Could you check a few things on this model? Use its own coordinates, in mm. Give positions to 0.01 mm unless a question says otherwise; leave off trailing zeros. Loops run counter-clockwise (first coordinate to the right, second up) from the corner with the lowest first, then second, coordinate; pieces in that order, holes last.
1. Imagine slicing it at A-A (y = -4.5). Count the separate pieces of the cut face and the enclosed holes in it, plus the area to 3 significant figures.
2. For P1, Ø18, axis at x = 0, z = 185, coming from the +Y side, with a flat end and sliding along its axis, tell me the tip position at first contact or that it passes through.
3. Thinking about a two-plate mould opening in Z: for faces 1 (the cylindrical face through (-1.302, 0.858, 94.915)), 2 (the cylindrical face through (-2.17, 0.86, 275.24)), 3 (the flat face through (-1, 2, 890)), 4 (the flat face through (-1, 32.799, 444)), which applies, +Z half, -Z half, draft (parallel to the pull), parting line (faces both ways), or undercut?
4. I need wall thicknesses on line 1 along X through (y, z) = (5, 585); line 2 along Z through (x, y) = (-21.5, 29.5); line 3 along Z through (x, y) = (-32, -26.5). Which ranges of each line are inside material? Lowest first, please.
5. Imagine slicing it at B-B (z = 285). List the corners of the cut face in (x, y) for me.
```python
from build123d import *

# Parameters (mm, degrees)
F0_W     = 75
F0_H     = 63
F1_DEPTH = 890
F2_R     = 10
F3_DEPTH = 63.001
F4_SIZE  = 10


with BuildPart() as f1:
    # F0 (on Top) → F1 (new body)
    with BuildSketch(Plane.XY):
        with Locations((0, 1.299331)):
            Rectangle(F0_W, F0_H)
    extrude(amount=F1_DEPTH)

    # F2 (on face) → F3 (cut, through all)
    with BuildSketch(Plane.XZ.offset(30.200669)):
        with Locations((0, 85)):
            Circle(F2_R)
        with Locations((0, 185)):
            Circle(F2_R)
        with Locations((0, 285)):
            Circle(F2_R)
        with Locations((0, 385)):
            Circle(F2_R)
        with Locations((0, 485)):
            Circle(F2_R)
        with Locations((0, 585)):
            Circle(F2_R)
        with Locations((0, 685)):
            Circle(F2_R)
        with Locations((0, 785)):
            Circle(F2_R)
    extrude(amount=-F3_DEPTH, mode=Mode.SUBTRACT)

    # F4
    f4_edges = [f1.edges().sort_by_distance(p)[0] for p in [
        (0, 32.799331, 0),
        (-37.5, 1.299331, 0),
        (0, -30.200669, 0),
    ]]
    chamfer(f4_edges, length=F4_SIZE)


solid = f1.part
```
Derived:
1. separate pieces: 1
1. enclosed holes: 8
1. area: 64,200 mm2
2. P1: passes through
3. face 1: undercut
3. face 2: undercut
3. face 3: +Z half
3. face 4: draft
4. line 1: x = -37.5 to -10, 10 to 37.5
4. line 2: z = 6.7 to 890
4. line 3: z = 6.3 to 890
5. outline: (-37.5, -30.2) - (-10, -30.2) - (-10, 32.8) - (-37.5, 32.8) - close; (10, -30.2) - (37.5, -30.2) - (37.5, 32.8) - (10, 32.8) - close
